CAD build for the part. Positions are in the model's coordinates, mm. Face numbers are marked on the shaded views. A direction names the side the tool comes from. Round coordinates to 2 decimals unless told otherwise and drop trailing zeros. Loops run counter-clockwise (first coordinate to the right, second up) from the corner with the lowest first, then second, coordinate; pieces in that order, holes last.
from build123d import *

# Parameters (mm, degrees)
SKETCH_1_R             = 20.1
EXTRUDE_1_DEPTH        = 68.2
SKETCH_2_R             = 5
CUT_EXTRUDE_1_DEPTH    = 2
SKETCH_3_R             = 2.5
EXTRUDE_2_DEPTH        = 20
CUT_EXTRUDE_START      = -15
CUT_EXTRUDE_2_DEPTH    = 15
CHAMFER_1_SIZE         = 1
M3X0_51_D              = 2.5
M3X0_51_DEPTH          = 8.5
M3X0_51_TIP            = 0.751075774
CUT_EXTRUDE_START_2    = -2.8
CUT_EXTRUDE_3_DEPTH    = 2.8
CHAMFER_2_SIZE         = 0.5
EXTRUDE_START          = 0.5
EXTRUDE_5_DEPTH        = 9
EXTRUDE_6_REACH        = 110.208
EXTRUDE_6_START_RADIUS = 20.1
EXTRUDE_6_END_RADIUS   = 20.1
SKETCH_10_W            = 7
SKETCH_10_H            = 18.5


# Read off the part's stored shape, not the designer's step: the extrude step
with BuildPart() as part:
    # Sketch 1 → Extrude 1 (new body)
    with BuildSketch(Plane.XY):
        Circle(SKETCH_1_R)
    extrude(amount=EXTRUDE_1_DEPTH)

    # Sketch 2 → Cut-Extrude 1 (cut)
    with BuildSketch(Plane.XY.offset(68.2)):
        Circle(SKETCH_2_R)
    extrude(amount=-CUT_EXTRUDE_1_DEPTH, mode=Mode.SUBTRACT)

    # Sketch 3 → Extrude 2 (add)
    with BuildSketch(Plane.XY.offset(66.2)):
        Circle(SKETCH_3_R)
    extrude(amount=EXTRUDE_2_DEPTH)

    # Sketch 4 → Cut-Extrude 2 (cut)
    with BuildSketch(Plane.XY.offset(86.2).offset(CUT_EXTRUDE_START)):
        with BuildLine():
            Line((2.1, 1.356465997), (2.1, -1.356465997))
            ThreePointArc((2.1, -1.356465997), (2.5, 0), (2.1, 1.356465997))
        make_face()
    extrude(amount=CUT_EXTRUDE_2_DEPTH, mode=Mode.SUBTRACT)

    # Chamfer 1
    chamfer_1_edges = [part.edges().sort_by_distance(p)[0] for p in [
        (-20.1, 0, 68.2),
    ]]
    chamfer(chamfer_1_edges, length=CHAMFER_1_SIZE)

    # M3x0.51
    with Locations(Plane.XY.offset(68.2)):
        with Locations((-10.825317547, 6.25), (0, 12.5), (10.825317547, 6.25), (10.825317547, -6.25), (0, -12.5), (-10.825317547, -6.25)):
            Hole(M3X0_51_D / 2, depth=M3X0_51_DEPTH)
            with Locations((0, 0, -(M3X0_51_DEPTH + M3X0_51_TIP / 2))):  # 118° drill point
                Cone(0, M3X0_51_D / 2, M3X0_51_TIP, mode=Mode.SUBTRACT)

    # Sketch 8 → Cut-Extrude 3 (cut)
    with BuildSketch(Plane.XY.offset(68.2).offset(CUT_EXTRUDE_START_2)):
        with BuildLine():
            Line((-14.212846302, 10.677312396), (-15.870249004, 12.334715098))
            ThreePointArc((-15.870249004, 12.334715098), (-14.212846302, 14.212846302), (-12.334715098, 15.870249004))
            Line((-12.334715098, 15.870249004), (-10.677312396, 14.212846302))
            ThreePointArc((-10.677312396, 14.212846302), (-10.677312396, 10.677312396), (-14.212846302, 10.677312396))
        make_face()
        with BuildLine():
            Line((14.212846302, 10.677312396), (15.870249004, 12.334715098))
            ThreePointArc((15.870249004, 12.334715098), (14.212846302, 14.212846302), (12.334715098, 15.870249004))
            Line((12.334715098, 15.870249004), (10.677312396, 14.212846302))
            ThreePointArc((10.677312396, 14.212846302), (10.677312396, 10.677312396), (14.212846302, 10.677312396))
        make_face()
        with BuildLine():
            Line((10.677312396, -14.212846302), (12.334715098, -15.870249004))
            ThreePointArc((12.334715098, -15.870249004), (14.212846302, -14.212846302), (15.870249004, -12.334715098))
            Line((15.870249004, -12.334715098), (14.212846302, -10.677312396))
            ThreePointArc((14.212846302, -10.677312396), (10.677312396, -10.677312396), (10.677312396, -14.212846302))
        make_face()
        with BuildLine():
            Line((-14.212846302, -10.677312396), (-15.870249004, -12.334715098))
            ThreePointArc((-15.870249004, -12.334715098), (-14.212846302, -14.212846302), (-12.334715098, -15.870249004))
            Line((-12.334715098, -15.870249004), (-10.677312396, -14.212846302))
            ThreePointArc((-10.677312396, -14.212846302), (-10.677312396, -10.677312396), (-14.212846302, -10.677312396))
        make_face()
    extrude(amount=CUT_EXTRUDE_3_DEPTH, mode=Mode.SUBTRACT)

    # Chamfer 2
    chamfer_2_edges = [part.edges().sort_by_distance(p)[0] for p in [
        (-20.1, 0, 0),
    ]]
    chamfer(chamfer_2_edges, length=CHAMFER_2_SIZE)

    # Extrude 5 outline → Extrude 5 (add)
    with BuildSketch(Plane.XY.offset(EXTRUDE_START)):
        with BuildLine():
            ThreePointArc((18.139428229, -10.5), (21.1, 0), (18.139428229, 10.5))
            Line((18.139428229, 10.5), (17.139428229, 10.5))
            ThreePointArc((17.139428229, 10.5), (20.1, 0), (17.139428229, -10.5))
            Line((17.139428229, -10.5), (18.139428229, -10.5))
        make_face()
    extrude(amount=EXTRUDE_5_DEPTH)

    # Extrude 6: from a cylinder face, 110.208 long prism both ways, kept between that surface and its translate by the depth
    extrude_6_start = Plane(origin=(1, 0, 5), z_dir=(0, 0, -1)) * Cylinder(EXTRUDE_6_START_RADIUS, 261.616, mode=Mode.PRIVATE)
    extrude_6_end = Plane(origin=(7.5, 0, 5), z_dir=(0, 0, -1)) * Cylinder(EXTRUDE_6_END_RADIUS, 261.616, mode=Mode.PRIVATE)
    # Sketch 10 → Extrude 6 (add, from a surface)
    with BuildSketch(Plane(origin=(30, 0, 0), x_dir=(0, 0, -1), z_dir=(1, 0, 0)), mode=Mode.PRIVATE) as extrude_6_sk1:
        with Locations((-5, 0)):
            Rectangle(SKETCH_10_W, SKETCH_10_H)
    extrude_6_tool1 = extrude(extrude_6_sk1.sketch, amount=EXTRUDE_6_REACH, both=True, mode=Mode.PRIVATE)
    add(((extrude_6_tool1 - extrude_6_start) & extrude_6_end).solids().sort_by_distance((22.095097, 0, 5))[0])


solid = part.part
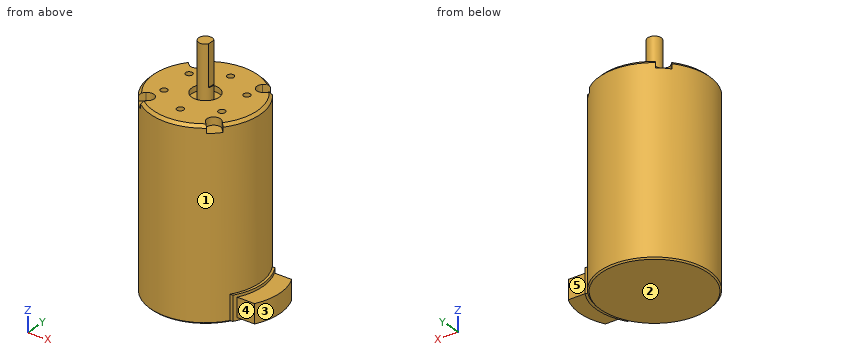
Item 1: Cut at B-B (y = 0). List the corners of the cut face in (x, z).
Verdict:
outline: (-20.1, 0.5) - (-19.6, 0) - (19.6, 0) - (20.1, 0.5) - (21.1, 0.5) - (21.1, 1.5) - (27.6, 1.5) - (27.6, 8.5) - (21.1, 8.5) - (21.1, 9.5) - (20.1, 9.5) - (20.1, 67.2) - (19.1, 68.2) - (5, 68.2) - (5, 66.2) - (2.5, 66.2) - (2.5, 71.2) - (2.1, 71.2) - (2.1, 86.2) - (-2.5, 86.2) - (-2.5, 66.2) - (-5, 66.2) - (-5, 68.2) - (-19.1, 68.2) - (-20.1, 67.2) - close
Item 2: Flat gauge pins, fed straight in: P1, Ø1.1, axis at x = 17.5, z = 4, coming from the -Y side; P2, Ø2, axis at x = -7.5, z = 23, coming from the +Y side; P3, Ø2, axis at y = 4.5, z = 61, coming from the -X side. Where does each tip first touch, or does it go through?
Verdict:
P1: stops at y = -10.8
P2: stops at y = 19.02
P3: stops at x = -19.79
Item 3: 3-axis set-ups, long thin cutter, end or side, ignore diameter. For the marked faces 1, 2, 3, 4 and 5: which of +Z, -Z, +X, -X, +Y, -Y reach the whole face in a straight line?
Verdict:
face 1: +Z
face 2: -Z, +X, -X, +Y, -Y
face 3: +Z, -Z, +X
face 4: +Z, -Z, +X, -Y
face 5: +Z, -Z, +X, +Y
Item 4: Wall check: L1, parallel to Z at x = 3, y = 11.5; L2, parallel to Z at x = -3, y = -0.5; L3, parallel to X at y = -6, z = 64. Give the ranges that are in metal, low to high.
Verdict:
L1: z = 0 to 68.2
L2: z = 0 to 66.2
L3: x = -19.18 to -12.05, -9.6 to 9.6, 12.05 to 19.18
Item 5: Cut at C-C (x = 23). List the corners of the cut face in (y, z).
Verdict:
outline: (-9.25, 1.5) - (9.25, 1.5) - (9.25, 8.5) - (-9.25, 8.5) - close
Item 6: Cut at A-A (z = 64). List the corners of the cut face in (x, y), plus the area to 3 significant figures.
Verdict:
outline: circle Ø40.2 at (0, 0); hole circle Ø2.5 at (-10.83, -6.25); hole circle Ø2.5 at (-10.83, 6.25); hole circle Ø2.5 at (0, -12.5); hole circle Ø2.5 at (0, 12.5); hole circle Ø2.5 at (10.83, -6.25); hole circle Ø2.5 at (10.83, 6.25)
area: 1,240 mm2
